```python
from build123d import *

# Parameters (mm, degrees)
SKETCH1_R           = 1.275
BOSS_EXTRUDE1_DEPTH = 5
SKETCH2_W           = 9.1
SKETCH2_H           = 17.8
BOSS_EXTRUDE2_DEPTH = 20
BOSS_EXTRUDE3_DEPTH = 3
CUT_EXTRUDE1_DEPTH  = 15
SKETCH5_R           = 2.5
CUT_EXTRUDE2_DEPTH  = 15
SKETCH7_W           = 24.2
SKETCH7_H           = 42.2
BOSS_EXTRUDE4_DEPTH = 5
SKETCH8_R           = 12
CUT_EXTRUDE3_DEPTH  = 5


with BuildPart() as part:
    # Sketch1 → Boss-Extrude1 (new body)
    # profile 1 of 2: a face of its own
    with BuildSketch(Plane(origin=(0, 0, 0), x_dir=(0, 0, -1), z_dir=(1, 0, 0))):
        Polygon((-4.381647728, -34.17856484), (-0.382647728, -30.17956484), (-0.382647728, 8.02143516), (-6.482647728, 8.02143516), (-9.382647728, 8.02143516), (-9.382647728, -34.17856484), align=None)
        with Locations((-5.982647728, 2.42143516)):
            Circle(SKETCH1_R, mode=Mode.SUBTRACT)
        with Locations((-5.982647728, -28.57856484)):
            Circle(SKETCH1_R, mode=Mode.SUBTRACT)
    # profile 2 of 2: a face of its own
    with BuildSketch(Plane(origin=(0, 0, 0), x_dir=(0, 0, -1), z_dir=(1, 0, 0))):
        Polygon((2.617352272, 8.02143516), (2.617352272, 25.82143516), (-6.482647728, 25.82143516), (-6.482647728, 8.02143516), (-0.382647728, 8.02143516), align=None)
    extrude(amount=BOSS_EXTRUDE1_DEPTH)

    # Sketch2 → Boss-Extrude2 (add)
    with BuildSketch(Plane(origin=(5, 0, 0), x_dir=(0, 0, -1), z_dir=(1, 0, 0))):
        with Locations((-1.932647728, 16.92143516)):
            Rectangle(SKETCH2_W, SKETCH2_H)
    extrude(amount=BOSS_EXTRUDE2_DEPTH)

    # Sketch3 → Boss-Extrude3 (add)
    with BuildSketch(Plane(origin=(0, 0, 0.382647728), x_dir=(-1, 0, 0), z_dir=(0, 0, -1))):
        Polygon((-25, 8.02143516), (0, 8.02143516), (0, -30.17956484), (-5, -30.17956484), align=None)
    extrude(amount=BOSS_EXTRUDE3_DEPTH)

    # Sketch4 → Cut-Extrude1 (cut, symmetric)
    with BuildSketch(Plane(origin=(5, 0, 0), x_dir=(0, 0, -1), z_dir=(1, 0, 0))):
        Polygon((-0.382647728, -30.17956484), (2.617352272, -27.17956484), (2.617352272, -30.17956484), align=None)
    extrude(amount=CUT_EXTRUDE1_DEPTH, both=True, mode=Mode.SUBTRACT)

    # Sketch5 → Cut-Extrude2 (cut, symmetric)
    with BuildSketch(Plane(origin=(0, 0, -2.617352272), x_dir=(-1, 0, 0), z_dir=(0, 0, -1))):
        with Locations((-19.86272871, 16.92143516)):
            Circle(SKETCH5_R)
    extrude(amount=CUT_EXTRUDE2_DEPTH, both=True, mode=Mode.SUBTRACT)


with BuildPart() as body_2:
    # Mirror14: mirrored copy
    add(part.part.mirror(Plane.XY.offset(21.482647728)))


with BuildPart() as part_1:
    add(part.part)

    add(body_2.part)  # Boss-Extrude4 merges body 2
    # Sketch7 → Boss-Extrude4 (add)
    with BuildSketch(Plane(origin=(5, 0, 0), x_dir=(0, 0, -1), z_dir=(1, 0, 0))):
        with Locations((-21.482647728, -13.07856484)):
            Rectangle(SKETCH7_W, SKETCH7_H)
    extrude(amount=-BOSS_EXTRUDE4_DEPTH)

    # Sketch8 → Cut-Extrude3 (cut)
    with BuildSketch(Plane(origin=(5, 0, 0), x_dir=(0, 0, -1), z_dir=(1, 0, 0))):
        with Locations((-21.482647728, -13.07856484)):
            Circle(SKETCH8_R)
    extrude(amount=-CUT_EXTRUDE3_DEPTH, mode=Mode.SUBTRACT)


solid = part_1.part
```
Here's how the part is built. I have some questions about the finished solid (model axes, mm). A direction names the side the tool comes from. Give positions to 0.01 mm unless a question says otherwise; leave off trailing zeros. Loops run counter-clockwise (first coordinate to the right, second up) from the corner with the lowest first, then second, coordinate; pieces in that order, holes last. Notation, with made-up numbers: (50, 69.25) -> (72, 69.25) arc R22 cw to (72, 82.25) -> close; hole circle Ø9 at (48.5, 85.5). An arc over 180 degrees is marked (long way). Use one line per item in the form item = value. Start each with the question number.
1) Thinking about a two-plate mould opening in Z: for faces 4 (the face through (12, 25.821, 2)), 5 (the face through (15, 8.021, 3)), 6 (the face through (2.6, -30.73, 42.03)), which applies, +Z half, -Z half, draft (parallel to the pull), parting line (faces both ways), or undercut?
2) Please list where these lines run through material, in increasing order: line 1 along Z through (x, y) = (13.75, 20); line 2 along Z through (x, y) = (15.5, 7.5); line 3 along Y through (x, z) = (13.25, 2.5).
3) Imagine slicing it at A-A (z = 25.5). Please give me the cut outline in (x, y).
4) Imagine slicing it at C-C (x = 20.5). Please give me the cut outline in (y, z).
5) Which directions (+Z, -Z, +X, -X, +Y, -Y) give clear straight access to the entire face, cutting with the end or side of a thin tool? Please do faces 1 (the face through (5, -3, 31)), 2 (the face through (3, 8.021, 22)), 3 (the face through (3, -34.179, 22)).
6) Imagine slicing it at B-B (y = -16.5). Please give me the cut outline in (x, z), then the cut area to 3 significant figures.
7) For P1, Ø4, axis at y = 2.42, z = 5.98, coming from the +X side; P2, Ø3, axis at y = -28.58, z = 36.98, coming from the -X side; P3, Ø6, axis at x = 18, z = 5.5, coming from the -Y side; P4, Ø1.5, axis at x = 2, z = 21, coming from the +Y side, each with a flat end and sliding along its axis, tell me the tip position at first contact or that it passes through.
8) Imagine slicing it at D-D (x = 11.5). Please give me the cut outline in (y, z).
Check values:
q1.face_4 = draft
q1.face_5 = undercut
q1.face_6 = +Z half
q2.line_1 = -2.62 to 6.48, 36.48 to 45.58
q2.line_2 = -2.62 to 0.38, 42.58 to 45.58
q2.line_3 = 8.02 to 25.82
q3.outline = (0, -34.18) -> (5, -34.18) -> (5, -24.39) -> (0, -24.39) -> close; (0, -1.77) -> (5, -1.77) -> (5, 8.02) -> (0, 8.02) -> close
q4.outline = (-0.57, -2.62) -> (14.5, -2.62) -> (14.5, 6.48) -> (8.02, 6.48) -> (8.02, 0.38) -> (-0.57, 0.38) -> close; (-0.57, 42.58) -> (8.02, 42.58) -> (8.02, 36.48) -> (14.5, 36.48) -> (14.5, 45.58) -> (-0.57, 45.58) -> close; (19.34, -2.62) -> (25.82, -2.62) -> (25.82, 6.48) -> (19.34, 6.48) -> close; (19.34, 36.48) -> (25.82, 36.48) -> (25.82, 45.58) -> (19.34, 45.58) -> close
q5.face_1 = +X, -Y
q5.face_2 = +X, -X, +Y
q5.face_3 = +Z, -Z, +X, -X, -Y
q6.outline = (0, -2.62) -> (12.16, -2.62) -> (12.16, 0.38) -> (5, 0.38) -> (5, 9.98) -> (0, 9.98) -> close; (0, 32.98) -> (5, 32.98) -> (5, 42.58) -> (12.16, 42.58) -> (12.16, 45.58) -> (0, 45.58) -> close
q6.area = 169 mm^2
q7.P1 = 5
q7.P2 = 0
q7.P3 = 8.02
q7.P4 = 8.02
q8.outline = (-17.76, -2.62) -> (25.82, -2.62) -> (25.82, 6.48) -> (8.02, 6.48) -> (8.02, 0.38) -> (-17.76, 0.38) -> close; (-17.76, 42.58) -> (8.02, 42.58) -> (8.02, 36.48) -> (25.82, 36.48) -> (25.82, 45.58) -> (-17.76, 45.58) -> close
